Input: part model. Units: mm. Frame: model coordinates. Face numbers are marked on the shaded views. A direction names the side the tool comes from. Coordinates: 2 decimals unless noted, no trailing zeros. Loops run counter-clockwise (first coordinate to the right, second up) from the corner with the lowest first, then second, coordinate; pieces in that order, holes last.
Item 1: Section A-A on z = 3.5. Give the number of separate pieces and of enclosed holes in the cut face, and give its area (3 significant figures).
Item 2: Section C-C on y = 8.25. Return loops of the section in (x, z), and give its area (3 significant figures).
Item 3: Reachability of the marked faces 4 and 5 from +Z, -Z, +X, -X, +Y, -Y: full face, straight path, thin tool, end or side. Return the list, or none.
Item 4: Contact query for flat-ended pins moving along their axis: P1, Ø1.4, axis at y = 11.5, z = 4, coming from the +X side; P2, Ø1, axis at x = 11, z = 2.5, coming from the -Y side; P3, Ø1, axis at x = -5.5, z = 4.5, coming from the -Y side (3 decimals). Output: stop coordinate, or through.
Item 5: Pull-direction query (X, two-part tool) for the marked faces 1, 2 and 3; classes: released by +X, released by -X, zero draft, split by the parting line, or undercut.
Item 6: Ray query, line 1 along Y through (x, z) = (0, 4.5); line 2 along X through (y, z) = (1, 2); line 3 along Z through (x, y) = (-6, -3.25). Return the intervals inside material, ascending.
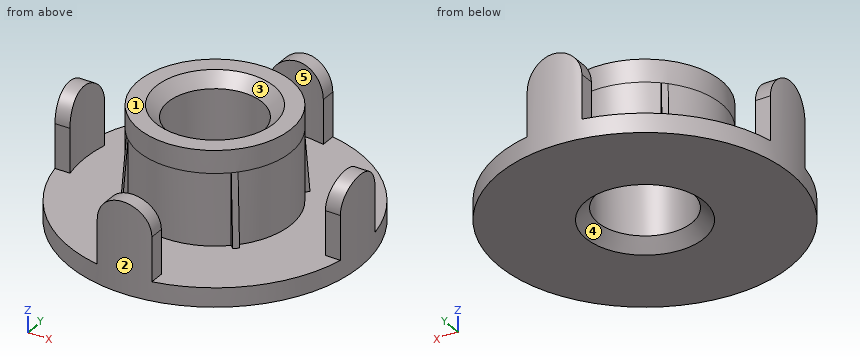
```python
from build123d import *

# Parameters (mm, degrees)
SKETCH_R           = 12.45
PAD_DEPTH          = 1.6
SKETCH001_R        = 6.4
PAD001_DEPTH       = 7.9
PAD002_DEPTH       = 14
POLARPATTERN_COUNT = 4
POCKET_DEPTH       = 10
SKETCH004_W        = 4
SKETCH004_H        = 10
SKETCH005_R        = 3.95
POCKET001_DEPTH    = 9.501
CHAMFER_SIZE       = 1


with BuildPart() as part:
    # Sketch → Pad (new body)
    with BuildSketch(Plane.XY):
        Circle(SKETCH_R)
    extrude(amount=PAD_DEPTH)

    # Sketch001 (on Face3 of Pad) → Pad001 (join)
    with BuildSketch(Plane.XY.offset(1.6)):
        Circle(SKETCH001_R)
    extrude(amount=PAD001_DEPTH)

    # Sketch002 → Pad002 (join)
    with BuildSketch(Plane.XZ):
        with BuildLine():
            Line((-2.3, 0), (-2.3, 5.3))
            ThreePointArc((2.3, 5.3), (0, 7.6), (-2.3, 5.3))
            Line((2.3, 0), (2.3, 5.3))
            Line((-2.3, 0), (2.3, 0))
        make_face()
    pad002 = extrude(amount=PAD002_DEPTH)

    # PolarPattern: Pad002 ×4 about axis
    polarpattern_axis = Axis((0, 0, 0), (0, 0, 1))
    for i in range(1, POLARPATTERN_COUNT):
        add(pad002.rotate(polarpattern_axis, i * 360 / POLARPATTERN_COUNT))

    # Sketch006 → Revolution (revolve)
    with BuildSketch(Plane.XZ):
        Polygon((0, 0), (0, 7.6), (6.4, 7.6), (7, 0), align=None)
    revolve(axis=Axis((0, 0, 0), (0, 0, 1)))

    # Sketch007 (on Face28 of Revolution) → Pocket (cut)
    with BuildSketch(Plane.XY.offset(1.6)):
        with BuildLine():
            ThreePointArc((-7.952942, 7.599389), (-11, 0), (-7.952942, -7.599389))
            Line((-7.952942, -7.599389), (-4.698806, -4.345253))
            ThreePointArc((-4.698806, 4.345253), (-6.4, 0), (-4.698806, -4.345253))
            Line((-7.952942, 7.599389), (-4.698806, 4.345253))
        make_face()
        with BuildLine():
            ThreePointArc((-7.599389, -7.952942), (0, -11), (7.599389, -7.952942))
            Line((7.599389, -7.952942), (4.345253, -4.698806))
            ThreePointArc((-4.345253, -4.698806), (0, -6.4), (4.345253, -4.698806))
            Line((-7.599389, -7.952942), (-4.345253, -4.698806))
        make_face()
        with BuildLine():
            ThreePointArc((7.952942, -7.599389), (11, 0), (7.952942, 7.599389))
            Line((7.952942, 7.599389), (4.698806, 4.345253))
            ThreePointArc((4.698806, -4.345253), (6.4, 0), (4.698806, 4.345253))
            Line((7.952942, -7.599389), (4.698806, -4.345253))
        make_face()
        with BuildLine():
            ThreePointArc((7.599389, 7.952942), (0, 11), (-7.599389, 7.952942))
            Line((-7.599389, 7.952942), (-4.345253, 4.698806))
            ThreePointArc((4.345253, 4.698806), (0, 6.4), (-4.345253, 4.698806))
            Line((7.599389, 7.952942), (4.345253, 4.698806))
        make_face()
    extrude(amount=POCKET_DEPTH, mode=Mode.SUBTRACT)

    # Sketch004 → Groove (revolve, cut)
    with BuildSketch(Plane.XZ):
        with Locations((-14.235706, 5)):
            Rectangle(SKETCH004_W, SKETCH004_H)
    revolve(axis=Axis((0, 0, 0), (0, 0, 1)), mode=Mode.SUBTRACT)

    # Sketch005 (on Face73 of Groove) → Pocket001 (cut, through all)
    with BuildSketch(Plane.XY.offset(9.5)):
        Circle(SKETCH005_R)
    extrude(amount=-POCKET001_DEPTH, mode=Mode.SUBTRACT)

    # Chamfer
    chamfer_edges = [part.edges().sort_by_distance(p)[0] for p in [
        (-3.95, 0, 9.5),
        (0, -3.95, 0),
    ]]
    chamfer(chamfer_edges, length=CHAMFER_SIZE)


solid = part.part
```
Results found:
1. separate pieces: 5
1. enclosed holes: 1
1. area: 103 mm2
2. outline: (-9.04, 0) - (9.04, 0) - (9.04, 1.6) - (-9.04, 1.6) - close
2. area: 28.9 mm2
3. face 4: -Z
3. face 5: +Z
4. P1: stops at x = 2.3
4. P2: stops at y = -2.3
4. P3: stops at y = -3.995
5. face 1: zero draft
5. face 2: split by the parting line
5. face 3: undercut
6. line 1: y = -12.24 to -11, -6.4 to -3.95, 3.95 to 6.4, 11 to 12.24
6. line 2: x = -12.19 to -10.95, -6.32 to -3.82, 3.82 to 6.32, 10.95 to 12.19
6. line 3: z = 0 to 1.6
